Check sheet for the modelled part. Datum: model origin and axes. Units: mm. Face numbers are marked on the shaded views. A direction names the side the tool comes from. Coordinates: 2 decimals unless noted, no trailing zeros. Write each loop counter-clockwise with the first axis right and the second up, starting at its lowest first coordinate (ties: lowest second). Pieces come first, ordered by that corner, then holes. Notation, with made-up numbers: (29, 16) -> (69, 16) arc R26 cw to (69, 52) -> close; hole circle Ø6 at (36, 3.5). An arc over 180 degrees is marked (long way). One line per item, written item: value. Start each with the question number.
1) Sectioned sample at B-B on x = 2.55. Enter the section's corners in (y, z), plus the area to 3 significant figures.
2) Sectioned sample at D-D on y = 16. Enter the section's corners in (x, z), plus the area to 3 significant figures.
3) Gauge pin test, flat ends, axial feed: P1, Ø2, axis at x = 3.5, y = -2.5, coming from the -Z side; P2, Ø3, axis at y = 3, z = -20, coming from the -X side; P3, Ø2.5, axis at x = 3, y = 21, coming from the -Z side; P4, Ø2.5, axis at x = 3.5, z = -7, coming from the -Y side. Record the tip position at first contact, or that the pin passes through.
4) Draft check along Y on the marked faces 3, 4, 5 and 6. Enter one of: +Y half, -Y half, draft (parallel to the pull), parting line (faces both ways), or undercut.
5) Set-up check for the marked faces 1 and 2: record each of +Z, -Z, +X, -X, +Y, -Y from which the full face is reachable in a straight line by a thin tool's end or side.
6) Scan lines: line 1 along Y through (x, z) = (3.8, -20); line 2 along Z through (x, y) = (3, 0.5); line 3 along Y through (x, z) = (4.2, -31.5). Record each from-to range of solid material in increasing order. Write a range as [from, to].
7) Sectioned sample at C-C on z = -20. Enter the section's corners in (x, y), plus the area to 3 significant figures.
8) Sectioned sample at A-A on z = -46.5. Enter the section's corners in (x, y).
```python
from build123d import *

# Parameters (mm, degrees)
SKETCH_1_W           = 55
SKETCH_1_H           = 45.45
SKETCH_1_W_2         = 40.2
SKETCH_1_H_2         = 20.7
EXTRUDE_1_DEPTH      = 5
SKETCH_2_W           = 30
SKETCH_2_H           = 4.8
EXTRUDE_2_DEPTH      = 5
SKETCH_3_R           = 1.1
CUT_EXTRUDE_1_DEPTH  = 5
FILLET_2_R           = 5
FILLET_3_R           = 1
M3_CLEARANCE_HOLE1_D = 3.4
SKETCH3_W            = 7.4
SKETCH3_H            = 20.7
CUT_EXTRUDE1_DEPTH   = 10
FILLET1_R            = 5


with BuildPart() as part:
    # 草图1 → 凸台-拉伸1 (new body)
    with BuildSketch(Plane(origin=(0, 0, 0), x_dir=(0, 0, -1), z_dir=(1, 0, 0))):
        with Locations((27.5, 22.725)):
            Rectangle(SKETCH_1_W, SKETCH_1_H)
        with Locations((27.5, 24)):
            Rectangle(SKETCH_1_W_2, SKETCH_1_H_2, mode=Mode.SUBTRACT)
    extrude(amount=EXTRUDE_1_DEPTH)

    # 草图2 → 凸台-拉伸2 (add)
    with BuildSketch(Plane.ZY):
        with Locations((-27.5, -2.4)):
            Rectangle(SKETCH_2_W, SKETCH_2_H)
    extrude(amount=-EXTRUDE_2_DEPTH)

    # 草图3 → 切除-拉伸1 (cut)
    with BuildSketch(Plane.ZY):
        with Locations((-42.5, 0)):
            Circle(SKETCH_3_R)
        with Locations((-12.5, 0)):
            Circle(SKETCH_3_R)
        with Locations((-7.4, 13.65)):
            Circle(SKETCH_3_R)
        with Locations((-7.4, 34.35)):
            Circle(SKETCH_3_R)
    extrude(amount=-CUT_EXTRUDE_1_DEPTH, mode=Mode.SUBTRACT)

    # 圆角2
    fillet_2_edges = [part.edges().sort_by_distance(p)[0] for p in [
        (2.5, 45.45, 0),
        (2.5, 45.45, -55),
        (2.5, 0, -55),
        (2.5, 0, 0),
    ]]
    fillet(fillet_2_edges, radius=FILLET_2_R)

    # 圆角3
    fillet_3_edges = [part.edges().sort_by_distance(p)[0] for p in [
        (2.5, -4.8, -42.5),
        (2.5, -4.8, -12.5),
    ]]
    fillet(fillet_3_edges, radius=FILLET_3_R)

    # M3 Clearance Hole1 (through all)
    with Locations(Plane.ZY):
        with Locations((-30, 3), (-20, 3)):
            Hole(M3_CLEARANCE_HOLE1_D / 2)

    # Sketch3 → Cut-Extrude1 (cut)
    with BuildSketch(Plane.ZY):
        with Locations((-51.3, 24)):
            Rectangle(SKETCH3_W, SKETCH3_H)
    extrude(amount=-CUT_EXTRUDE1_DEPTH, mode=Mode.SUBTRACT)

    # Fillet1
    fillet1_edges = [part.edges().sort_by_distance(p)[0] for p in [
        (2.5, 13.65, -55),
        (2.5, 34.35, -55),
    ]]
    fillet(fillet1_edges, radius=FILLET1_R)


solid = part.part
```
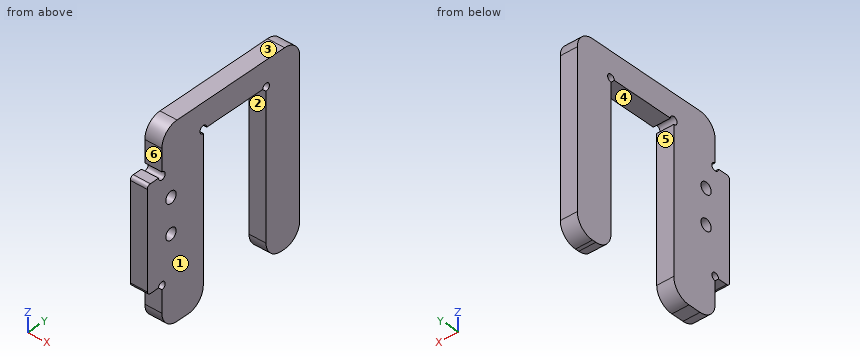
Answers:
1. outline: (-4.8, -41.5) arc R1 ccw to (-3.8, -42.5) -> (-1.1, -42.5) arc R1.1 cw (long way) to (0, -43.6) -> (0, -50) arc R5 ccw to (5, -55) -> (8.65, -55) arc R5 ccw to (13.65, -50) -> (13.65, -8.5) arc R1.1 cw (long way) to (14.75, -7.4) -> (33.25, -7.4) arc R1.1 cw (long way) to (34.35, -8.5) -> (34.35, -50) arc R5 ccw to (39.35, -55) -> (40.45, -55) arc R5 ccw to (45.45, -50) -> (45.45, -5) arc R5 ccw to (40.45, 0) -> (5, 0) arc R5 ccw to (0, -5) -> (0, -11.4) arc R1.1 cw (long way) to (-1.1, -12.5) -> (-3.8, -12.5) arc R1 ccw to (-4.8, -13.5) -> close; hole circle Ø3.4 at (3, -30); hole circle Ø3.4 at (3, -20)
1. area: 1,600 mm2
2. outline: (0, -7.4) -> (5, -7.4) -> (5, 0) -> (0, 0) -> close
2. area: 37.0 mm2
3. P1: stops at z = -42.5
3. P2: passes through
3. P3: stops at z = -7.4
3. P4: stops at y = 0
4. face 3: draft
4. face 4: undercut
4. face 5: undercut
4. face 6: -Y half
5. face 1: +Z, -Z, +X, +Y, -Y
5. face 2: -Z, +X, -X
6. line 1: y = [-4.8, 1.3], [4.7, 13.65], [34.35, 45.45]
6. line 2: z = [-52.18, -43.48], [-41.52, -13.48], [-11.52, -2.82]
6. line 3: y = [-4.8, 2.2], [3.8, 13.65], [34.35, 45.45]
7. outline: (0, -4.8) -> (5, -4.8) -> (5, 1.3) -> (0, 1.3) -> close; (0, 4.7) -> (5, 4.7) -> (5, 13.65) -> (0, 13.65) -> close; (0, 34.35) -> (5, 34.35) -> (5, 45.45) -> (0, 45.45) -> close
7. area: 131 mm2
8. outline: (0, 0) -> (5, 0) -> (5, 13.65) -> (0, 13.65) -> close; (0, 34.35) -> (5, 34.35) -> (5, 45.45) -> (0, 45.45) -> close
